Geometry: final body of the model. Coordinates: model frame, mm. Face numbers are marked on the shaded views. Round coordinates to 2 decimals unless told otherwise and drop trailing zeros. Loops run counter-clockwise (first coordinate to the right, second up) from the corner with the lowest first, then second, coordinate; pieces in that order, holes last. Notation, with made-up numbers: M 77.25,-36 L 102.25,-36 A10 cw 102.25,-24 Z; hole C 83,68.5 d2. An arc over 180 degrees is marked long. Write each question's results on one line, items separated by ' | '.
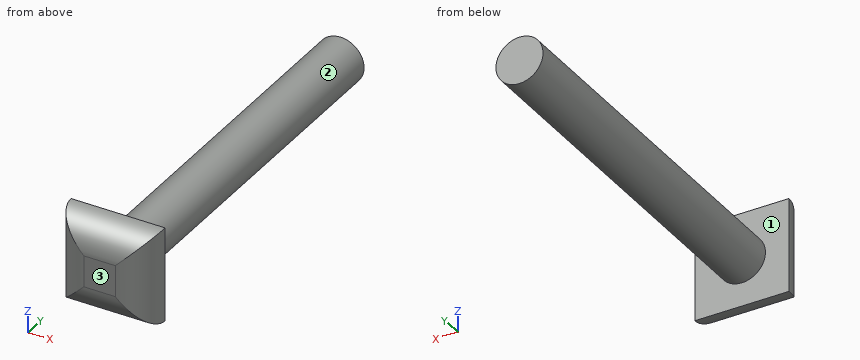
```python
from build123d import *

# Parameters (mm, degrees)
SKETCH1_W           = 24
SKETCH1_H           = 24
BOSS_EXTRUDE1_DEPTH = 8
SKETCH2_R           = 6
BOSS_EXTRUDE2_DEPTH = 96
FILLET1_R           = 8


with BuildPart() as part:
    # Sketch1 → Boss-Extrude1 (new body)
    with BuildSketch(Plane(origin=(0, 0, 0), x_dir=(1, 0, 0), z_dir=(0, 1, 0))):
        Rectangle(SKETCH1_W, SKETCH1_H)
    extrude(amount=BOSS_EXTRUDE1_DEPTH)

    # Sketch2 → Boss-Extrude2 (add)
    with BuildSketch(Plane(origin=(0, 8, 0), x_dir=(1, 0, 0), z_dir=(0, 1, 0))):
        with Locations(Location((0, 0, 0), (0, 0, 90))):
            Circle(SKETCH2_R)
    extrude(amount=BOSS_EXTRUDE2_DEPTH)

    # Fillet1
    fillet1_edges = [part.edges().sort_by_distance(p)[0] for p in [
        (0, 0, 12),
        (12, 0, 0),
        (-12, 0, 0),
        (0, 0, -12),
    ]]
    fillet(fillet1_edges, radius=FILLET1_R - 0.0001)  # a hair under: the kernel refuses the full size


solid = part.part
```
1. Section C-C (y = 23.5). Output: boundary loops of the cut face in (x, z), then the cut area to 3 significant figures.
Answer key:
outline: C 0,0 d12 | area: 113 mm²
2. Ray query, probe 1 along X at (y, z) = (77, -0.5); probe 2 along Y at (x, z) = (5.5, -1.25); probe 3 along Z at (x, y) = (-3.25, 99.5). Return the intervals inside material, ascending.
Answer key:
probe 1: x = -5.98 to 5.98 | probe 2: y = 0.14 to 104 | probe 3: z = -5.04 to 5.04
3. Pin query (flat end, axial travel): P1, Ø12, axis at y = 48.5, z = 9.5, coming from the +X side; P2, Ø6, axis at x = -3, z = 5, coming from the -Y side; P3, Ø2, axis at y = 10.5, z = -3, coming from the +X side; P4, Ø1.5, axis at x = -1.5, z = -9, coming from the +Y side. Return the tip coordinate at first contact, or that it passes through.
Answer key:
P1: stops at x = 4.87 | P2: stops at y = 0 | P3: stops at x = 5.66 | P4: stops at y = 8
4. Draft query along Y for the marked faces 1, 2 and 3. Return one class per face: pulls with the +Y half, pulls with the -Y half, needs draft (parallel to the pull), parting line crosses it, or undercut.
Answer key:
face 1: pulls with the +Y half | face 2: needs draft | face 3: pulls with the -Y half
